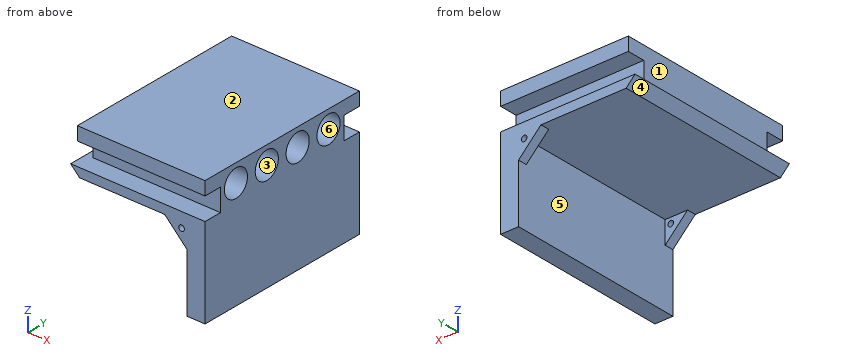
from build123d import *

# Parameters (mm, degrees)
SKETCH1_W           = 20
SKETCH1_H           = 40
BOSS_EXTRUDE1_DEPTH = 80
SKETCH8_W           = 16
SKETCH8_H           = 64
BOSS_EXTRUDE2_DEPTH = 57
SKETCH10_R          = 6
CUT_EXTRUDE1_DEPTH  = 51
SKETCH12_W          = 57
SKETCH12_H          = 6
BOSS_EXTRUDE3_DEPTH = 8
SKETCH14_W          = 57
SKETCH14_H          = 6
BOSS_EXTRUDE4_DEPTH = 8
SKETCH17_W          = 48
SKETCH17_H          = 80
CUT_EXTRUDE4_DEPTH  = 36
CHAMFER1_SIZE       = 10
SKETCH16_W          = 48
SKETCH16_H          = 72
CUT_EXTRUDE5_DEPTH  = 10
SKETCH19_R          = 1.25
CUT_EXTRUDE6_DEPTH  = 105.703357948


with BuildPart() as part:
    # Sketch1 → Boss-Extrude1 (new body)
    with BuildSketch(Plane(origin=(0, 0, 0), x_dir=(1, 0, 0), z_dir=(0, 1, 0))):
        Polygon((-17.351649908, 20.312727502), (-57.351649908, -19.687272498), (-17.351649908, -19.687272498), align=None)
        with Locations((-7.351649908, 0.312727502)):
            Rectangle(SKETCH1_W, SKETCH1_H)
    extrude(amount=-BOSS_EXTRUDE1_DEPTH)

    # Sketch8 → Boss-Extrude2 (add)
    with BuildSketch(Plane(origin=(2.648350092, 0, 0), x_dir=(0, 0, -1), z_dir=(1, 0, 0))):
        with Locations((-27.687272498, -40)):
            Rectangle(SKETCH8_W, SKETCH8_H)
    extrude(amount=-BOSS_EXTRUDE2_DEPTH)

    # Sketch10 → Cut-Extrude1 (cut)
    with BuildSketch(Plane(origin=(2.648350092, 0, 0), x_dir=(0, 0, -1), z_dir=(1, 0, 0))):
        with Locations((-27.687272498, -16)):
            Circle(SKETCH10_R)
        with Locations(Location((-27.687272498, -32, 0), (0, 0, 180))):
            Circle(SKETCH10_R)
        with Locations(Location((-27.687272498, -64, 0), (0, 0, 180))):
            Circle(SKETCH10_R)
        with Locations((-27.687272498, -48)):
            Circle(SKETCH10_R)
    extrude(amount=-CUT_EXTRUDE1_DEPTH, mode=Mode.SUBTRACT)

    # Sketch12 → Boss-Extrude3 (add)
    with BuildSketch(Plane.XZ.offset(72)):
        with Locations((-25.851649908, 32.687272498)):
            Rectangle(SKETCH12_W, SKETCH12_H)
    extrude(amount=BOSS_EXTRUDE3_DEPTH)

    # Sketch14 → Boss-Extrude4 (add)
    with BuildSketch(Plane(origin=(0, -8, 0), x_dir=(1, 0, 0), z_dir=(0, 1, 0))):
        with Locations((-25.851649908, -32.687272498)):
            Rectangle(SKETCH14_W, SKETCH14_H)
    extrude(amount=BOSS_EXTRUDE4_DEPTH)

    # Sketch17 → Cut-Extrude4 (cut)
    with BuildSketch(Plane(origin=(0, 0, -20.312727502), x_dir=(-1, 0, 0), z_dir=(0, 0, -1))):
        with Locations((29.351649908, -40)):
            Rectangle(SKETCH17_W, SKETCH17_H)
    extrude(amount=-CUT_EXTRUDE4_DEPTH, mode=Mode.SUBTRACT)

    # Chamfer1
    chamfer1_edges = [part.edges().sort_by_distance(p)[0] for p in [
        (-5.351649908, -40, 15.687272498),
    ]]
    chamfer(chamfer1_edges, length=CHAMFER1_SIZE)

    # Sketch16 → Cut-Extrude5 (cut)
    with BuildSketch(Plane(origin=(0, 0, 15.687272498), x_dir=(-1, 0, 0), z_dir=(0, 0, -1))):
        with Locations((29.351649908, -40)):
            Rectangle(SKETCH16_W, SKETCH16_H)
    extrude(amount=CUT_EXTRUDE5_DEPTH, mode=Mode.SUBTRACT)

    # Sketch19 → Cut-Extrude6 (cut, through all)
    with BuildSketch(Plane(origin=(0, 0, 0), x_dir=(1, 0, 0), z_dir=(0, 1, 0))):
        with Locations(Location((-7.851649908, -13.187272498, 0), (0, 0, 270))):
            Circle(SKETCH19_R)
    extrude(amount=-CUT_EXTRUDE6_DEPTH, mode=Mode.SUBTRACT)


solid = part.part
Design review of the part built by this model. Coordinates are the model's own, in mm. Face numbers are marked on the shaded views. A direction names the side the tool comes from. Round coordinates to 2 decimals unless told otherwise and drop trailing zeros. Loops run counter-clockwise (first coordinate to the right, second up) from the corner with the lowest first, then second, coordinate; pieces in that order, holes last. Notation, with made-up numbers: (2, 0.5) - (13, 0.5) arc R31 ccw to (13, 27.5) - close; hole circle Ø4 at (68, 49.25). An arc over 180 degrees is marked (long way). One line per item, written item: value. Start each with the question number.
1) For the marked faces 4, 5 and 6, list the 3-axis set-ups (+Z, -Z, +X, -X, +Y, -Y) from which the entire face can be reached by the end or side of a thin tool; tool diameter is ignored.
2) Consider section D-D on z = 3.5. Give the boundary of the cut face in (x, y), then the cut area to 3 significant figures.
3) Consider section C-C on x = -10.5. Give the boundary of the cut face in (y, z), then the cut area to 3 significant figures.
4) Draft analysis for pull direction Z (two halves, no side actions). For the marked faces 1, 2 and 3, state which applies: +Z half, -Z half, draft (parallel to the pull), parting line (faces both ways), or undercut.
5) To check wall thickness, follow L1, parallel to Y at x = -4, z = 29; L2, parallel to Z at x = -21, y = -5.5; L3, parallel to X at y = -38, z = 10. State the ranges of each line that lie inside material, in increasing order. Write a range as from..to.
6) Consider section A-A on x = -33. Give the boundary of the cut face in (y, z).
7) Insertion check: pin 1 Ø9 at (x, y) = (-37.5, -3.5) entering from -Z; pin 2 Ø6 at (y, z) = (-31, 26.5) entering from +X; pin 3 Ø11 at (y, z) = (-25, -4.5) entering from -X; pin 4 Ø11 at (x, z) = (-28, 24) entering from +Y. Each pin has a flat end and moves straight along its axis. Give the tip position at first contact, or say it passes through.
8) Consider section B-B on y = -16. Give the boundary of the cut face in (x, z), then the cut area to 3 significant figures.
Reported:
1. face 4: -Z, -X, +Y, -Y
1. face 5: -Z, -X
1. face 6: +X
2. outline: (-5.35, -80) - (2.65, -80) - (2.65, 0) - (-5.35, 0) - close
2. area: 640 mm^2
3. outline: (-80, 10.84) - (-76, 10.84) - (-76, 15.69) - (-4, 15.69) - (-4, 10.84) - (0, 10.84) - (0, 19.69) - (-8, 19.69) - (-8, 29.69) - (0, 29.69) - (0, 35.69) - (-80, 35.69) - (-80, 29.69) - (-72, 29.69) - (-72, 19.69) - (-80, 19.69) - close; hole circle Ø12 at (-64, 27.69); hole circle Ø12 at (-48, 27.69); hole circle Ø12 at (-32, 27.69); hole circle Ø12 at (-16, 27.69)
3. area: 1,030 mm^2
4. face 1: draft
4. face 2: +Z half
4. face 3: undercut
5. L1: y = -72..-69.85, -58.15..-53.85, -42.15..-37.85, -26.15..-21.85, -10.15..-8
5. L2: z = 15.69..19.69, 29.69..35.69
5. L3: x = -5.35..2.65
6. outline: (-80, 15.69) - (0, 15.69) - (0, 19.69) - (-8, 19.69) - (-8, 29.69) - (0, 29.69) - (0, 35.69) - (-80, 35.69) - (-80, 29.69) - (-72, 29.69) - (-72, 19.69) - (-80, 19.69) - close; hole circle Ø12 at (-64, 27.69); hole circle Ø12 at (-48, 27.69); hole circle Ø12 at (-32, 27.69); hole circle Ø12 at (-16, 27.69)
7. pin 1: stops at z = 15.69
7. pin 2: stops at x = -48.35
7. pin 3: stops at x = -5.35
7. pin 4: stops at y = 0
8. outline: (-57.35, 19.69) - (-53.35, 15.69) - (-5.35, 15.69) - (-5.35, -20.31) - (2.65, -20.31) - (2.65, 21.69) - (-48.35, 21.69) - (-48.35, 33.69) - (2.65, 33.69) - (2.65, 35.69) - (-54.35, 35.69) - (-54.35, 19.69) - close
8. area: 820 mm^2
